Design review of the part built by this model. Coordinates are the model's own, in mm. Face numbers are marked on the shaded views. A direction names the side the tool comes from. Give positions to 0.01 mm unless a question says otherwise; leave off trailing zeros. Loops run counter-clockwise (first coordinate to the right, second up) from the corner with the lowest first, then second, coordinate; pieces in that order, holes last. Notation, with made-up numbers: M -10.75,1 L 44.25,1 A25 ccw 44.25,32 Z; hole C -16.75,0.25 d9. An arc over 180 degrees is marked long. Use CSV: the item, a comma, the result in double quotes.
Autodesk Inventor part; units mm, degrees
ref_plane "YZ Plane" through (0, 0, 0) normal (1, 0, 0) x (0, 1, 0)
ref_plane "XZ Plane" through (0, 0, 0) normal (0, 1, 0) x (-1, 0, 0)
ref_plane "XY Plane" through (0, 0, 0) normal (0, 0, 1) x (1, 0, 0)
sketch "Sketch1" plane through (0, 0, 0) normal (0, 1, 0) x (-1, 0, 0)
  line L0 (-1.7321, -3) -> (-3.4641, 0)
  line L1 (-3.4641, 0) -> (-1.7321, 3)
  line L2 (-1.7321, 3) -> (1.7321, 3)
  line L3 (1.7321, 3) -> (3.4641, 0)
  line L4 (3.4641, 0) -> (1.7321, -3)
  line L5 (1.7321, -3) -> (-1.7321, -3)
  point P0 (0, 0)
  point P1 (0, 0)
  point P2 (0, 0)
  dimension "d0" = 3
extrude "Extrusion1" add sketch "Sketch1" along normal blind 20
hole "Hole2" at (0, 0, 0) direction (0, 1, 0) diameter 3.242 depth 11.8 tip angle 118
sketch "Sketch3" plane through (0, 20, 0) normal (0, 1, 0) x (1, 0, 0)
  circle A0 centre (0, 0) radius 2
  dimension "d17" = 4
extrude "Extrusion2" add sketch "Sketch3" along normal blind 6
thread "Thread1"
chamfer "Chamfer1" distance 0.7 angle 45 1 edges at (-2, 26, 0)
properties part number "StandoffM4x20B" material "Brass, Soft Yellow"
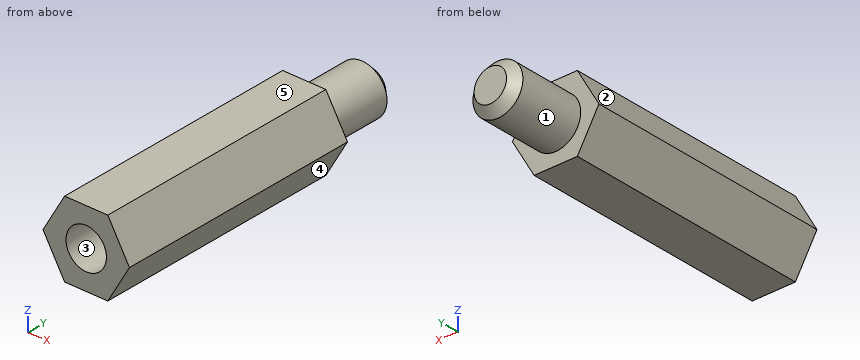
(1) Clearance check with flat-ended pins moving along their axes: P1, Ø3, axis at x = 0, z = 0, coming from the -Y side; P2, Ø1, axis at y = 22, z = -2, coming from the +X side. State where each tip first meets the part, or that it passes through.
A:
P1,"y = 11.87"
P2,"x = 1.32"
(2) We need section A-A on y = 3. State the section outline as (x, z) points, then the cut area to 3 significant figures.
A:
outline,"M -3.46,0 L -1.73,-3 L 1.73,-3 L 3.46,0 L 1.73,3 L -1.73,3 Z; hole C 0,0 d3.24"
area,"22.9 mm²"
(3) We need section C-C on z = -2.6. State the section outline as (x, y) points.
A:
outline,"M -1.96,0 L 1.96,0 L 1.96,20 L -1.96,20 Z"
(4) We need section D-D on x = 2.25. State the section outline as (y, z) points, then the cut area to 3 significant figures.
A:
outline,"M 0,-2.1 L 20,-2.1 L 20,2.1 L 0,2.1 Z"
area,"84.1 mm²"
(5) The part is to be moulded in two halves that separate along Z. For the marked faces 3, 4 and 5, say which applies: released by +Z, released by -Z, zero draft, split by the parting line, or undercut.
A:
face 3,"undercut"
face 4,"released by -Z"
face 5,"released by +Z"
(6) We need section B-B on y = 19. State the section outline as (x, z) points, then the cut area to 3 significant figures.
A:
outline,"M -3.46,0 L -1.73,-3 L 1.73,-3 L 3.46,0 L 1.73,3 L -1.73,3 Z"
area,"31.2 mm²"
(7) Wall thickness on line 1 along Z through (x, y) = (0, 9.25); line 2 along Y through (x, z) = (-1.25, 1.95); line 3 along X through (y, z) = (10.75, -0.8): over which ranges is each line inside the solid? List them lowest first. Write a range as [from, to].
A:
line 1,"[-3, -1.62], [1.62, 3]"
line 2,"[0, 20]"
line 3,"[-3, -1.41], [1.41, 3]"
(8) Machinability: for the marked faces 1 and 2, which of the approach directions +Z, -Z, +X, -X, +Y, -Y give a long, thin tool a straight path to every point of the face, cutting with its end or side? Answer none if there is none.
A:
face 1,"+Y"
face 2,"+Z, -X, +Y, -Y"
